```python
from build123d import *

# Parameters (mm, degrees)
BOSS_EXTRUDE1_DEPTH = 10
CUT_EXTRUDE1_DEPTH  = 40.884332764
SKETCH5_W           = 6
SKETCH5_H           = 3.5
BOSS_EXTRUDE2_DEPTH = 6
SKETCH2_R           = 2.95
SKETCH2_R_2         = 1.5
BOSS_EXTRUDE3_DEPTH = 4


with BuildPart() as part:
    # Sketch1 → Boss-Extrude1 (new, symmetric)
    with BuildSketch(Plane.YZ):
        Polygon((-20.35, 5.9), (-27.6, 5.9), (-27.6, 8.4), (-20.35, 8.4), (-20.35, 18.6), (20.35, 18.6), (20.35, 8.4), (27.6, 8.4), (27.6, 5.9), (20.35, 5.9), (20.35, -18.6), (-20.35, -18.6), align=None)
    extrude(amount=BOSS_EXTRUDE1_DEPTH, both=True)

    # Sketch4 → Cut-Extrude1 (cut, through all)
    with BuildSketch(Plane.XY.offset(8.4)):
        with BuildLine():
            Line((-6, -25.707050808), (-6, -27.6))
            Line((-6, -27.6), (-4, -27.6))
            Line((-4, -27.6), (-4, -25.707050808))
            ThreePointArc((-4, -25.707050808), (-5, -21.975), (-6, -25.707050808))
        make_face()
        with BuildLine():
            Line((6, -27.6), (4, -27.6))
            Line((4, -27.6), (4, -25.707050808))
            ThreePointArc((4, -25.707050808), (5, -21.975), (6, -25.707050808))
            Line((6, -25.707050808), (6, -27.6))
        make_face()
    cut_extrude1 = extrude(amount=-CUT_EXTRUDE1_DEPTH, mode=Mode.SUBTRACT)

    # Mirror1: Cut-Extrude1 across plane
    add(cut_extrude1.mirror(Plane.ZX), mode=Mode.SUBTRACT)

    # Sketch5 → Boss-Extrude2 (add)
    with BuildSketch(Plane.XZ.offset(20.35)):
        with Locations((0, -14.85)):
            Rectangle(SKETCH5_W, SKETCH5_H)
    extrude(amount=BOSS_EXTRUDE2_DEPTH)

    # Sketch2 → Boss-Extrude3 (add)
    with BuildSketch(Plane.XY.offset(18.6)):
        with Locations(Location((0, -10.35, 0), (0, 0, 180))):
            Circle(SKETCH2_R)
        with Locations((0, -10.35)):
            Circle(SKETCH2_R_2, mode=Mode.SUBTRACT)
    extrude(amount=BOSS_EXTRUDE3_DEPTH)


solid = part.part
```
Design review of the part built by this model. Coordinates are the model's own, in mm. A direction names the side the tool comes from. Coordinates: 2 decimals unless noted, no trailing zeros. Order: outer loops, then holes, each group sorted by start corner. A loop starts at its lowest first (then second) coordinate and runs counter-clockwise, first axis right, second up.
1) Take a section at C-C, the plane z = 3.5. Give the boundary of the cut face in (x, y), and give its area (3 significant figures).
2) Clearance check with flat-ended pins moving along their axes: pin 1 (1 mm diameter, centred on x = 4, z = -6, fed in from -Y); pin 2 (8 mm diameter, centred on x = -1.5, y = -24.5, fed in from +Z); pin 3 (6.5 mm diameter, centred on x = -5, y = 23.975, fed in from -Z); pin 4 (3.5 mm diameter, centred on x = 5, y = 23.975, fed in from -Z). State where each tip first meets the part, or that it passes through.
3) Mouldability with a two-part tool opening along Z and no side actions: class faces 1 (the flat face through (0, 24, 8.4)), 2 (the flat face through (0, -24, 5.9)), 3 (the flat face through (0, 27.6, 7)), 4 (the flat face through (0, 0, -18.6)) as +Z half, -Z half, draft (parallel to the pull), parting line (faces both ways), or undercut.
4) Take a section at D-D, the plane x = 5. Give the boundary of the cut face in (y, z) (3 decimals), and give its area (3 significant figures).
5) Take a section at B-B, the plane y = -1.5. Give the boundary of the cut face in (x, z), and give its area (3 significant figures).
6) Wall thickness on line 1 along Y through (x, z) = (0, 20); line 2 along Z through (x, y) = (-1.75, 20); line 3 along Y through (x, z) = (9, -2.5): over which ranges is each line inside the solid? List them lowest first.
7) For faces 5 (the flat face through (-4, -27, 7)), 6 (the flat face through (0, 20.35, -6)), 7 (the flat face through (3, -23, -15)), 8 (the cylindrical face through (-4.927, -21.976, 7.168)), list the 3-axis set-ups (+Z, -Z, +X, -X, +Y, -Y) from which the entire face can be reached by the end or side of a thin tool; tool diameter is ignored.
8) Take a section at A-A, the plane x = 0. Give the boundary of the cut face in (y, z), and give its area (3 significant figures).
Returned:
1. outline: (-10, -20.35) - (10, -20.35) - (10, 20.35) - (-10, 20.35) - close
1. area: 814 mm2
2. pin 1: stops at y = -20.35
2. pin 2: stops at z = 8.4
2. pin 3: stops at z = 5.9
2. pin 4: passes through
3. face 1: +Z half
3. face 2: undercut
3. face 3: draft
3. face 4: -Z half
4. outline: (-21.975, 5.9) - (-20.35, 5.9) - (-20.35, -18.6) - (20.35, -18.6) - (20.35, 5.9) - (21.975, 5.9) - (21.975, 8.4) - (20.35, 8.4) - (20.35, 18.6) - (-20.35, 18.6) - (-20.35, 8.4) - (-21.975, 8.4) - close
4. area: 1,520 mm2
5. outline: (-10, -18.6) - (10, -18.6) - (10, 18.6) - (-10, 18.6) - close
5. area: 744 mm2
6. line 1: y = -13.3 to -11.85, -8.85 to -7.4
6. line 2: z = -18.6 to 18.6
6. line 3: y = -20.35 to 20.35
7. face 5: +Z, -Z, -Y
7. face 6: -Z, +X, -X, +Y
7. face 7: -Z, +X, -Y
7. face 8: +Z, -Z
8. outline: (-27.6, 5.9) - (-20.35, 5.9) - (-20.35, -13.1) - (-26.35, -13.1) - (-26.35, -16.6) - (-20.35, -16.6) - (-20.35, -18.6) - (20.35, -18.6) - (20.35, 5.9) - (27.6, 5.9) - (27.6, 8.4) - (20.35, 8.4) - (20.35, 18.6) - (-7.4, 18.6) - (-7.4, 22.6) - (-8.85, 22.6) - (-8.85, 18.6) - (-11.85, 18.6) - (-11.85, 22.6) - (-13.3, 22.6) - (-13.3, 18.6) - (-20.35, 18.6) - (-20.35, 8.4) - (-27.6, 8.4) - close
8. area: 1,580 mm2
